Geometry: see drawing. Coordinates: mm, zero at the bounding-box minimum. A direction names the side the tool comes from. Give positions to 0.01 mm unless a question says otherwise; leave off trailing zeros. Loops run counter-clockwise (first coordinate to the right, second up) from the corner with the lowest first, then second, coordinate; pieces in that order, holes last. Notation, with made-up numbers: (19.5, 62.5) -> (25.5, 62.5) arc R26 cw to (25.5, 99.5) -> close; hole circle Ø3 at (-26, 18.5). An arc over 180 degrees is marked (long way). Use CSV: the item, a comma, the result in double quotes.
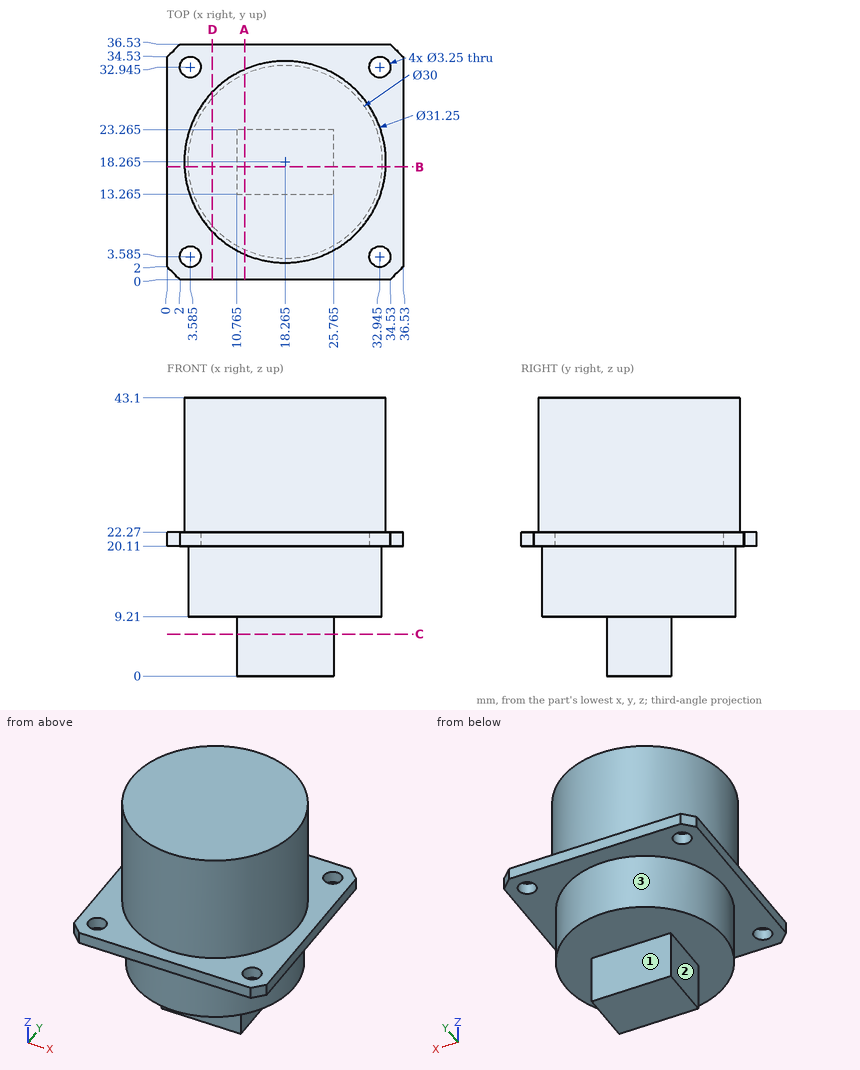
1) Section query D-D (x = 7). Return loops of the section in (y, z).
From the geometry:
outline,"(0, 20.11) -> (8.36, 20.11) -> (8.36, 9.21) -> (28.17, 9.21) -> (28.17, 20.11) -> (36.53, 20.11) -> (36.53, 22.27) -> (29.09, 22.27) -> (29.09, 43.1) -> (7.44, 43.1) -> (7.44, 22.27) -> (0, 22.27) -> close"
2) Section query B-B (y = 17.5). Return loops of the section in (x, z) (3 decimals), then the cut area to 3 significant figures.
From the geometry:
outline,"(0, 20.11) -> (3.285, 20.11) -> (3.285, 9.21) -> (10.765, 9.21) -> (10.765, 0) -> (25.765, 0) -> (25.765, 9.21) -> (33.245, 9.21) -> (33.245, 20.11) -> (36.53, 20.11) -> (36.53, 22.27) -> (33.871, 22.27) -> (33.871, 43.1) -> (2.659, 43.1) -> (2.659, 22.27) -> (0, 22.27) -> close"
area,"1,190 mm^2"
3) Contact query for flat-ended pins moving along their axis: pin 1 (7.5 mm diameter, centred on x = 18.5, z = 5.5, fed in from -Y) (3 decimals); pin 2 (1 mm diameter, centred on x = 11, z = 10, fed in from -Y); pin 3 (10 mm diameter, centred on x = 19.5, z = 4.5, fed in from +Y) (3 decimals); pin 4 (8 mm diameter, centred on x = 4, z = 21, fed in from -Y). Output: stop coordinate, or through.
From the geometry:
pin 1,"stops at y = 3.265"
pin 2,"stops at y = 4.88"
pin 3,"stops at y = 33.265"
pin 4,"stops at y = 0"
4) Section query C-C (z = 6.5). Return loops of the section in (x, y) (3 decimals).
From the geometry:
outline,"(10.765, 13.265) -> (25.765, 13.265) -> (25.765, 23.265) -> (10.765, 23.265) -> close"
5) Reachability of the marked faces 1, 2 and 3 from +Z, -Z, +X, -X, +Y, -Y: full face, straight path, thin tool, end or side. Return the list, or none.
From the geometry:
face 1,"-Z, +X, -X, +Y"
face 2,"-Z, -X, +Y, -Y"
face 3,"-Z"
6) Ray query, line 1 (Z direction, x = 19, y = 8); line 2 (Z direction, x = 29, y = 31); line 3 (X direction, y = 18, z = 9) (3 decimals). Return the intervals inside material, ascending.
From the geometry:
line 1,"z = 9.21 to 43.1"
line 2,"z = 20.11 to 22.27"
line 3,"x = 10.765 to 25.765"
7) Section query A-A (x = 12). Return loops of the section in (y, z) (3 decimals), then the cut area to 3 significant figures.
From the geometry:
outline,"(0, 20.11) -> (4.636, 20.11) -> (4.636, 9.21) -> (13.265, 9.21) -> (13.265, 0) -> (23.265, 0) -> (23.265, 9.21) -> (31.894, 9.21) -> (31.894, 20.11) -> (36.53, 20.11) -> (36.53, 22.27) -> (32.579, 22.27) -> (32.579, 43.1) -> (3.951, 43.1) -> (3.951, 22.27) -> (0, 22.27) -> close"
area,"1,060 mm^2"
